Can you work these out from the drawing? Everything is in mm from the part's minimum corner. A direction names the side the tool comes from. Coordinates: 2 decimals unless noted, no trailing zeros. Loops run counter-clockwise (first coordinate to the right, second up) from the corner with the lowest first, then second, coordinate; pieces in that order, holes last.
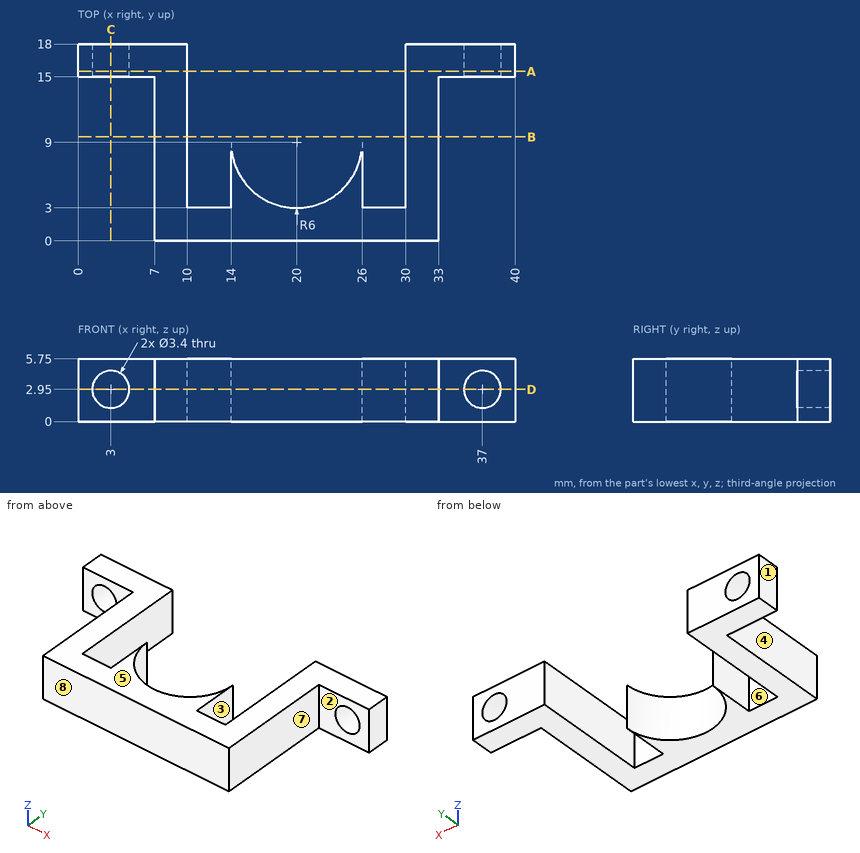
1) For the marked faces 4, 5, 6, 7 and 8, which set-ups out of +Z, -Z, +X, -X, +Y, -Y let a thin tool reach every point of the face, with its end or its side?
2) Will these pins go through, and if not, where does the flat tip stop? pin 1 (2 mm diameter, centred on y = 3.5, z = 3, fed in from -X); pin 2 (3 mm diameter, centred on y = 6, z = 4.5, fed in from +X); pin 3 (3 mm diameter, centred on x = 37, z = 2.5, fed in from -Y); pin 4 (3 mm diameter, centred on x = 26, y = 2.5, fed in from -Z).
3) If I drill on L1, parallel to X at y = 17.2, z = 2.95; L2, parallel to X at y = 9.5, z = 4.65; L3, parallel to Z at x = 37, y = 15.9, over which ranges is the centre line in solid material (lowest first)?
4) We'd pull the mould along X, two halves only. Please class the marked faces 1, 2 and 3: released by +X, released by -X, zero draft, split by the parting line, or undercut.
5) Imagine slicing it at C-C on x = 3. List the corners of the cut face in (y, z) for me, plus the area to 3 significant figures.
6) Imagine slicing it at A-A on y = 15.5. List the corners of the cut face in (x, z) for me, plus the area to 3 significant figures.
7) Imagine slicing it at D-D on z = 2.95. List the corners of the cut face in (x, y) for me, plus the area to 3 significant figures.
8) Imagine slicing it at B-B on y = 9.5. List the corners of the cut face in (x, z) for me, plus the area to 3 significant figures.
Solved:
1. face 4: +Z, -Z, -X, -Y
1. face 5: +Z, +X, -X, +Y, -Y
1. face 6: +Z, -Z, +Y
1. face 7: +Z, -Z, +X, -Y
1. face 8: +Z, -Z, +X, -X, -Y
2. pin 1: stops at x = 7
2. pin 2: stops at x = 33
2. pin 3: stops at y = 15
2. pin 4: stops at z = 0
3. L1: x = 0 to 1.3, 4.7 to 10, 30 to 35.3, 38.7 to 40
3. L2: x = 7 to 10, 30 to 33
3. L3: z = 0 to 1.25, 4.65 to 5.75
4. face 1: released by -X
4. face 2: zero draft
4. face 3: undercut
5. outline: (15, 0) - (18, 0) - (18, 1.25) - (15, 1.25) - close; (15, 4.65) - (18, 4.65) - (18, 5.75) - (15, 5.75) - close
5. area: 7.05 mm2
6. outline: (0, 0) - (10, 0) - (10, 5.75) - (0, 5.75) - close; (30, 0) - (40, 0) - (40, 5.75) - (30, 5.75) - close; hole circle Ø3.4 at (3, 2.95); hole circle Ø3.4 at (37, 2.95)
6. area: 96.8 mm2
7. outline: (0, 15) - (1.3, 15) - (1.3, 18) - (0, 18) - close; (4.7, 15) - (7, 15) - (7, 0) - (33, 0) - (33, 15) - (35.3, 15) - (35.3, 18) - (30, 18) - (30, 3) - (26, 3) - (26, 9) arc R6 cw to (14, 9) - (14, 3) - (10, 3) - (10, 18) - (4.7, 18) - close; (38.7, 15) - (40, 15) - (40, 18) - (38.7, 18) - close
7. area: 205 mm2
8. outline: (7, 0) - (10, 0) - (10, 5.75) - (7, 5.75) - close; (30, 0) - (33, 0) - (33, 5.75) - (30, 5.75) - close
8. area: 34.5 mm2
